Answer from the drawing. Dimensions are ordinates in mm from the lowest x, y and z of the part. Coordinates: 2 decimals unless noted, no trailing zeros. Order: outer loops, then holes, each group sorted by start corner. A loop starts at its lowest first (then second) coordinate and runs counter-clockwise, first axis right, second up.
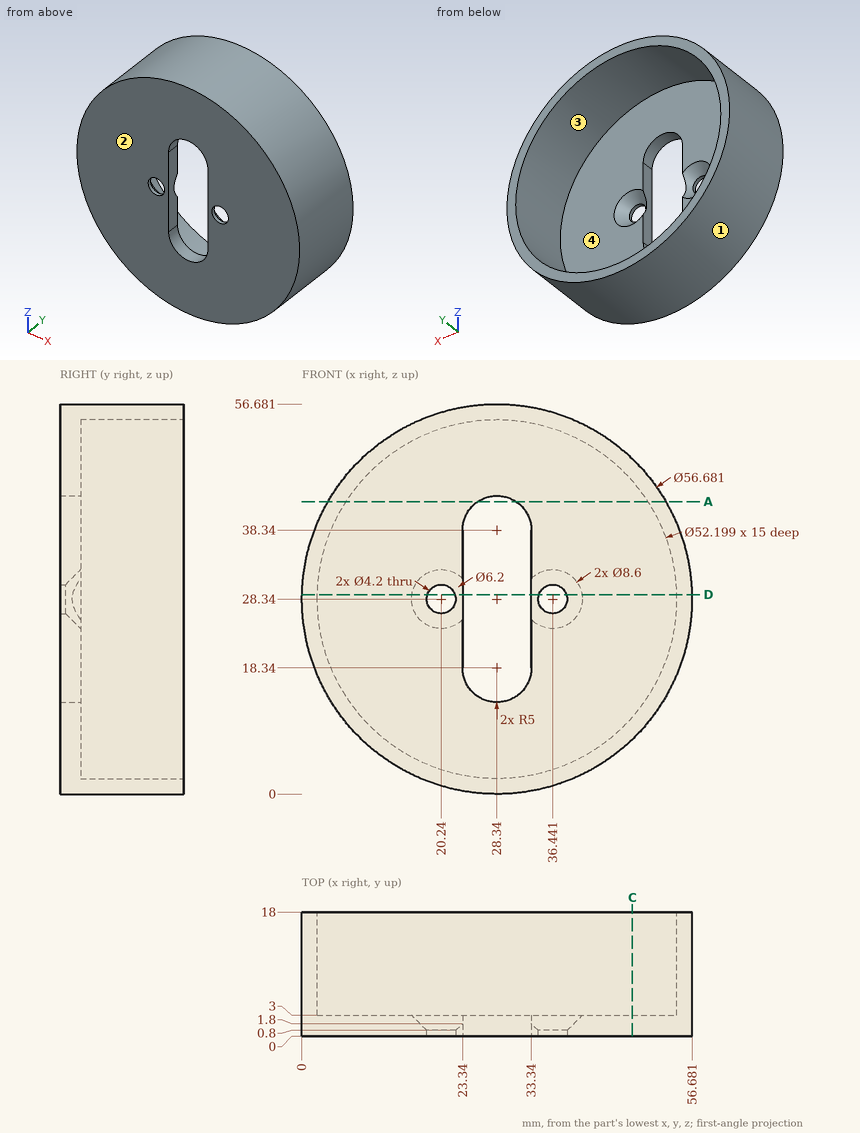
1) Each of these flat-tipped pins is pushed along its axis until it touches: P1, Ø6, axis at y = 13.5, z = 14, coming from the -X side; P2, Ø2, axis at x = 28, y = 11, coming from the -Z side; P3, Ø5, axis at y = 14, z = 40, coming from the +X side; P4, Ø2.5, axis at x = 20.24, z = 28.34, coming from the +Y side. Where does it stop, or does it pass through?
2) Determine the mould class of the marked faces 1, 2, 3 and 4 for opening direction X: released by +X, released by -X, zero draft, split by the parting line, or undercut.
3) Section D-D (z = 29) is taken. Give the number of separate pieces and of enclosed holes in the cut face.
4) Section A-A (z = 42.5) is taken. Give the vertices of the cut face in (x, y) (1 decimal).
5) Consider L1, parallel to X at y = 5.5, z = 29; L2, parallel to Y at x = 42, z = 29.5; L3, parallel to X at y = 1.75, z = 37 (1 decimal). Determine where each line is inside the solid, lowest interval first.
6) Section C-C (x = 48) is taken. Give the vertices of the cut face in (y, z) (1 decimal).
Filled sheet:
1. P1: stops at x = 2.37
1. P2: stops at z = 0
1. P3: stops at x = 55.16
1. P4: passes through
2. face 1: split by the parting line
2. face 2: zero draft
2. face 3: undercut
2. face 4: undercut
3. separate pieces: 4
3. enclosed holes: 0
4. outline: (3.8, 0) - (25.6, 0) - (25.6, 3) - (6.4, 3) - (6.4, 18) - (3.8, 18) - close; (31.1, 0) - (52.9, 0) - (52.9, 18) - (50.3, 18) - (50.3, 3) - (31.1, 3) - close
5. L1: x = 0.01 to 2.25, 54.43 to 56.67
5. L2: y = 0 to 3
5. L3: x = 1.4 to 23.3, 33.3 to 55.3
6. outline: (0, 7.9) - (18, 7.9) - (18, 11.2) - (3, 11.2) - (3, 45.5) - (18, 45.5) - (18, 48.8) - (0, 48.8) - close
